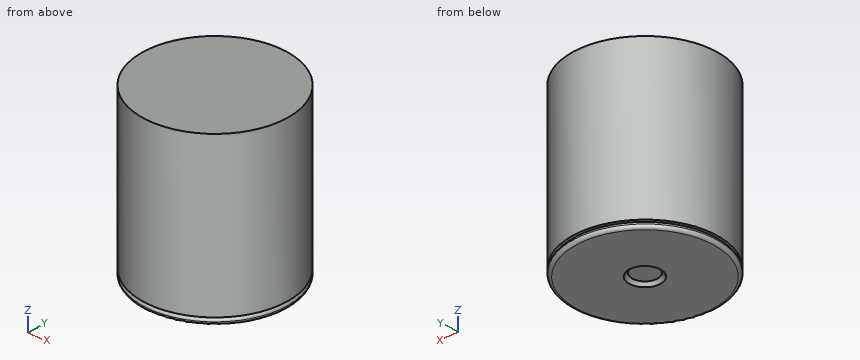
```python
from build123d import *

# Parameters (mm, degrees)
SKETCH_1_R          = 11.5
EXTRUDE_1_DEPTH     = 25
SKETCH_2_R          = 7.5
EXTRUDE_2_DEPTH     = 0.1
EXTRUDE_START       = 1
SKETCH_3_R          = 11.5
EXTRUDE_3_DEPTH     = 1
FILLET_1_R          = 0.5
FILLET_2_R          = 0.5
SKETCH_4_R          = 2.5
CUT_EXTRUDE_1_DEPTH = 0.5
CHAMFER_1_SIZE      = 0.5


# Some blends are built 0.0001 mm under size
with BuildPart() as part:
    # 草图1 → 凸台-拉伸1 (new body)
    with BuildSketch(Plane.XY):
        Circle(SKETCH_1_R)
    extrude(amount=EXTRUDE_1_DEPTH)

    # 草图2 → 凸台-拉伸2 (add)
    with BuildSketch(Plane(origin=(0, 0, 0), x_dir=(-1, 0, 0), z_dir=(0, 0, -1))):
        Circle(SKETCH_2_R)
    extrude(amount=EXTRUDE_2_DEPTH)

    # 草图3 → 凸台-拉伸3 (add)
    with BuildSketch(Plane(origin=(0, 0, -0.1), x_dir=(-1, 0, 0), z_dir=(0, 0, -1)).offset(EXTRUDE_START)):
        with Locations(Location((0, 0, 0), (0, 0, 180))):
            Circle(SKETCH_3_R)
    extrude(amount=-EXTRUDE_3_DEPTH)

    # 圆角1
    fillet_1_edges = [part.edges().sort_by_distance(p)[0] for p in [
        (-11.5, 0, -1.1),
    ]]
    fillet(fillet_1_edges, radius=FILLET_1_R)

    # 圆角2
    # the kernel refuses this fillet: 0.5 mm, written as the material it adds along each edge
    with BuildSketch(Plane(origin=(0, 0, -0.1), x_dir=(-1, 0, 0), z_dir=(0, -1, 0))) as fillet_2_piece_1:
        with BuildLine():
            CenterArc((7.8, -0.5), FILLET_2_R, 90, 36.869897646)
            Line((7.5, -0.1), (7.5, 0))
            Line((7.5, 0), (7.8, 0))
        make_face()
    revolve(axis=Axis((0, 0, -0.1), (0, 0, -1)))
    # the kernel refuses this fillet: 0.5 mm, written as the material it takes off along each edge
    with BuildSketch(Plane(origin=(0, 0, -0.1), x_dir=(1, 0, 0), z_dir=(0, 1, 0))) as fillet_2_2_piece_1:
        with BuildLine():
            CenterArc((11.5 - FILLET_2_R, FILLET_2_R), FILLET_2_R, 270, 90)
            Line((11.5 - FILLET_2_R, 0), (11.5, 0))
            Line((11.5, 0), (11.5, FILLET_2_R))
        make_face()
    revolve(axis=Axis((0, 0, -0.1), (0, 0, -1)), mode=Mode.SUBTRACT)

    # 草图4 → 切除-拉伸1 (cut)
    with BuildSketch(Plane(origin=(0, 0, -1.1), x_dir=(-1, 0, 0), z_dir=(0, 0, -1))):
        Circle(SKETCH_4_R)
    extrude(amount=-CUT_EXTRUDE_1_DEPTH, mode=Mode.SUBTRACT)

    # 倒角1
    chamfer_1_edges = [part.edges().sort_by_distance(p)[0] for p in [
        (2.5, 0, -0.6),
    ]]
    chamfer(chamfer_1_edges, length=CHAMFER_1_SIZE - 0.0001)  # a hair under: the kernel refuses the full size


solid = part.part
```
Part model, mm, in its own coordinate system. Round coordinates to 2 decimals unless told otherwise and drop trailing zeros. Order: outer loops, then holes, each group sorted by start corner. A loop starts at its lowest first (then second) coordinate and runs counter-clockwise, first axis right, second up. Notation, with made-up numbers: M -15.75,62.25 L -9.75,62.25 A31 ccw -9.75,96.25 Z; hole C 12.5,14 d9. An arc over 180 degrees is marked long. Answer in a Markdown table with one row per item. Add a question column.
Q1. Wall check: L1, parallel to Y at x = 0, z = 6.5; L2, parallel to X at y = 3.75, z = 3.5; L3, parallel to Y at x = 4.5, z = 18.5. Give the ranges that are in metal, low to high. Write a range as from..to.
Q2. Pin check, flat tips, straight feed: pin 1 (2 mm diameter, centred on y = 1.5, z = 9.5, fed in from -X); pin 2 (1.2 mm diameter, centred on x = -0.5, y = -0.5, fed in from -Z); pin 3 (12 mm diameter, centred on y = -8.5, z = 16.5, fed in from +X) (3 decimals). Stop position of each tip, or through.
Q3. Cut at A-A on z = 20.5. Give the cut face in (x, y).
Established:
| question | item | result |
|---|---|---|
| 1 | L1 | y = -11.5..11.5 |
| 1 | L2 | x = -10.87..10.87 |
| 1 | L3 | y = -10.58..10.58 |
| 2 | pin 1 | stops at x = -11.49 |
| 2 | pin 2 | stops at z = -0.6 |
| 2 | pin 3 | stops at x = 11.225 |
| 3 | outline | C 0,0 d23 |
